Geometry: final body of the model. Coordinates: model frame, mm. Face numbers are marked on the shaded views. A direction names the side the tool comes from. Give positions to 0.01 mm unless a question says otherwise; leave off trailing zeros. Loops run counter-clockwise (first coordinate to the right, second up) from the corner with the lowest first, then second, coordinate; pieces in that order, holes last.
1. Section A-A, the plane y = 0. Output: boundary loops of the cut face in (x, z), then the cut area to 3 significant figures.
2. Section C-C, the plane y = -32.5. Output: boundary loops of the cut face in (x, z).
3. Access query for the marked faces 5 and 6. Directions: +Z, -Z, +X, -X, +Y, -Y. A direction counts if a zero-diameter tool reaches every point of the face in a straight line with its end or side. Return the directions, or none.
4. Material intervals for line 1 along Y through (x, z) = (0, 7.75); line 2 along Y through (x, z) = (48.5, 7); line 3 along Y through (x, z) = (45.5, -5), sorted ascending.
5. First-contact query: P1, Ø5, axis at y = 78.5, z = 7, coming from the +X side; P2, Ø6, axis at y = 26, z = -11.5, coming from the -X side; P3, Ø12, axis at y = -47, z = -3, coming from the -X side. Flat tips, straight axial feed; report the tip coordinate or a pass-through.
6. Draft query along X for the marked faces 1, 2, 3 and 4. Return one class per face: +X half, -X half, draft (parallel to the pull), parting line (faces both ways), or undercut.
7. Section D-D, the plane x = -34.5. Output: boundary loops of the cut face in (y, z).
8. Section B-B, the plane x = -84. Output: boundary loops of the cut face in (y, z).
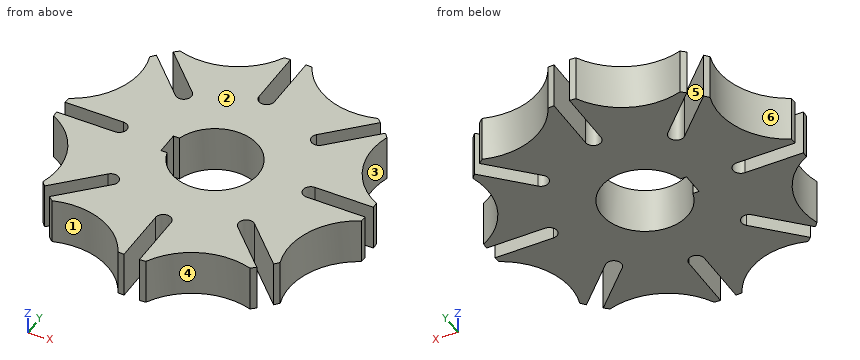
from build123d import *

# Parameters (mm, degrees)
SKETCH1_R           = 100
BOSS_EXTRUDE1_DEPTH = 15
CUT_EXTRUDE2_START  = -30
CUT_EXTRUDE2_DEPTH  = 30
CIRPATTERN1_COUNT   = 8
CUT_EXTRUDE3_DEPTH  = 30
CIRPATTERN2_COUNT   = 8
CUT_EXTRUDE4_DEPTH  = 35


# Read off the part's stored shape, not the designer's step: Cut-Extrude2
with BuildPart() as part:
    # Sketch1 → Boss-Extrude1 (new, symmetric)
    with BuildSketch(Plane.XY):
        Circle(SKETCH1_R)
    extrude(amount=BOSS_EXTRUDE1_DEPTH, both=True)

    # Cut-Extrude2 outline → Cut-Extrude2 (cut)
    with BuildSketch(Plane.XY.offset(15).offset(CUT_EXTRUDE2_START)):
        with BuildLine():
            ThreePointArc((62, 5), (57, 0), (62, -5))
            Line((62, -5), (99.874921777, -5))
            ThreePointArc((99.874921777, -5), (100, 0), (99.874921777, 5))
            Line((99.874921777, 5), (62, 5))
        make_face()
    cut_extrude2 = extrude(amount=CUT_EXTRUDE2_DEPTH, mode=Mode.SUBTRACT)

    # CirPattern1: Cut-Extrude2 ×8 about axis
    cirpattern1_axis = Axis((0, 0, 15), (0, 0, -1))
    for i in range(1, CIRPATTERN1_COUNT):
        add(cut_extrude2.rotate(cirpattern1_axis, i * 360 / CIRPATTERN1_COUNT), mode=Mode.SUBTRACT)

    # Sketch8 → Cut-Extrude3 (cut)
    with BuildSketch(Plane.XY.offset(15)):
        with BuildLine():
            ThreePointArc((76.781373425, 64.06731378), (78.062131756, 32.338894345), (99.594176537, 9))
            ThreePointArc((99.594176537, 9), (92.386069934, 38.27288965), (76.781373425, 64.06731378))
        make_face()
    cut_extrude3 = extrude(amount=-CUT_EXTRUDE3_DEPTH, mode=Mode.SUBTRACT)

    # CirPattern2: Cut-Extrude3 ×8 about axis
    cirpattern2_axis = Axis((0, 0, 0), (0, 0, 1))
    for i in range(1, CIRPATTERN2_COUNT):
        add(cut_extrude3.rotate(cirpattern2_axis, i * 360 / CIRPATTERN2_COUNT), mode=Mode.SUBTRACT)

    # Sketch9 → Cut-Extrude4 (cut, symmetric)
    with BuildSketch(Plane.XY.offset(15)):
        with BuildLine():
            Line((-26.97684192, 7.5), (-30.97684192, 7.5))
            Line((-30.97684192, 7.5), (-30.97684192, -7.5))
            Line((-30.97684192, -7.5), (-26.97684192, -7.5))
            ThreePointArc((-26.97684192, -7.5), (28, 0), (-26.97684192, 7.5))
        make_face()
    extrude(amount=CUT_EXTRUDE4_DEPTH, both=True, mode=Mode.SUBTRACT)


solid = part.part
Answers below:
1. outline: (-57, -15) - (-30.98, -15) - (-30.98, 15) - (-57, 15) - close; (28, -15) - (57, -15) - (57, 15) - (28, 15) - close
1. area: 1,650 mm2
2. outline: (-78, -15) - (78, -15) - (78, 15) - (-78, 15) - close
3. face 5: +Z, -Z
3. face 6: +Z, -Z, -X
4. line 1: y = -57 to -28, 28 to 57
4. line 2: y = -74.58 to -55.57, -41.43 to 41.43, 55.57 to 74.59
4. line 3: y = -74.77 to -52.57, -39.12 to 39.12, 52.57 to 74.78
5. P1: stops at x = 64.99
5. P2: stops at x = -83.27
5. P3: stops at x = -75.44
6. face 1: undercut
6. face 2: draft
6. face 3: +X half
6. face 4: undercut
7. outline: (-77.23, -15) - (77.23, -15) - (77.23, 15) - (-77.23, 15) - close
8. outline: (-22.03, -15) - (-5, -15) - (-5, 15) - (-22.03, 15) - close; (5, -15) - (22.02, -15) - (22.02, 15) - (5, 15) - close
